Source: CAD feature listing. Evaluate the final solid. Frame: model axes, mm. A direction names the side the tool comes from. Give positions to 0.01 mm unless a question says otherwise; leave off trailing zeros. Order: outer loops, then holes, each group sorted by start corner. A loop starts at its lowest first (then second) coordinate and runs counter-clockwise, first axis right, second up.
Autodesk Inventor part; units mm, degrees
ref_plane "YZ Plane" through (0, 0, 0) normal (1, 0, 0) x (0, 1, 0)
ref_plane "XZ Plane" through (0, 0, 0) normal (0, 1, 0) x (-1, 0, 0)
ref_plane "XY Plane" through (0, 0, 0) normal (0, 0, 1) x (1, 0, 0)
sketch "Sketch1" plane through (0, 0, 0) normal (0, 1, 0) x (-1, 0, 0)
  line L0 (0, 0) -> (-85, 0)
  line L1 (-85, 0) -> (-85, -51)
  line L2 (-85, -51) -> (0, -51)
  line L3 (0, -51) -> (0, 0)
  line L4 (10, -71) -> (-95, -71)
  line L5 (-95, -71) -> (-95, 10)
  line L6 (10, 10) -> (10, -71)
  line L7 (10, 10) -> (-95, 10)
  circle A0 centre (-88, -53.5) radius 1.5
  line L8 (-42.5, -71) -> (-42.5, 10) construction
  circle A1 centre (3, -53.5) radius 1.5
  line L9 (0, -25.5) -> (-85, -25.5) construction
  circle A2 centre (-88, 2.5) radius 1.5
  circle A3 centre (3, 2.5) radius 1.5
  dimension "d0" = 85
  dimension "d1" = 51
  dimension "d2" = 20
  dimension "d3" = 10
  dimension "d4" = 10
  dimension "d13" = 2.5
  dimension "d14" = 3
  dimension "d15" = 3
  dimension "d34" = 10
extrude "Extrusion1" add sketch "Sketch1" along normal blind 5
sketch "Sketch2" plane through (95, 0, 10) normal (1, 0, 0) x (0, 0, -1)
  line L0 (68, -22.5167) -> (68, 0) construction
  line L1 (82.1908, -7.9375) -> (94.6908, 13.7132)
  line L2 (0, 0) -> (81, 0) construction
  line L3 (81, 5) -> (81, 0)
  line L4 (94.6908, 13.7132) -> (90.3607, 16.2132)
  line L5 (90.3607, 16.2132) -> (81, 0)
  line L6 (68.4427, 0) -> (82.1908, -7.9375)
  line L7 (81, 0) -> (68.4427, 0)
  point P0 (10, 0)
  dimension "d16" = 30
  dimension "d18" = 13
  dimension "d26" = 5
  dimension "d33" = 45
  dimension "d37" = 25
extrude "Extrusion2" add sketch "Sketch2" against normal blind 105
sketch "Sketch3" plane through (95, -32.5167, -58) normal (0, -0.5, -0.866) x (-1, 0, 0)
  line L0 (7.5, 46.3816) -> (97.5, 46.3816) construction
  line L1 (7.5, 43.1316) -> (97.5, 43.1316)
  line L2 (97.5, 49.6316) -> (7.5, 49.6316)
  arc A0 (7.5, 49.6316) -> (7.5, 43.1316) centre (7.5, 46.3816) ccw
  arc A1 (97.5, 43.1316) -> (97.5, 49.6316) centre (97.5, 46.3816) ccw
  line L3 (0, 53.3816) -> (105, 53.3816) construction
  point P0 (95, -0.8397)
  point P1 (52.5, 46.3816)
  point P2 (52.5, 53.3816)
  point P3 (52.5, 53.3816)
  dimension "d21" = 6.5
  dimension "d22" = 90
  dimension "d23" = 7
extrude "Extrusion3" cut sketch "Sketch3" against normal through all
sketch "Sketch4" plane through (95, 0, 10) normal (1, 0, 0) x (0, 0, -1)
  line L0 (81, 0) -> (81, 5)
  line L1 (81, 0) -> (72, 5)
  line L2 (72, 5) -> (81, 5)
  line L3 (81, 5) -> (81, 0)
  point P0 (10, 0)
  dimension "d28" = 9
extrude "Extrusion4" cut sketch "Sketch4" against normal through all
fillet "Fillet3" radius 2 3 edges at (-10, 14.9632, -82.5257) (95, 14.9632, -82.5257) (42.5, 0, -71)
fillet "Fillet4" radius 2 1 edges at (42.5, -7.9375, -72.1908)
fillet "Fillet5" radius 2 2 edges at (42.5, 5, -62) (42.5, 0, -58.4427)
fillet "Fillet6" radius 2 2 edges at (-10, 2.5, 10) (95, 2.5, 10)
equation "\"d34\" = d4"
properties part number "screen mount"
1) Section query B-B on x = 53. Output: boundary loops of the cut face in (y, z).
Checks:
outline: (-6.94, -70.46) arc R2 ccw to (-6.21, -73.19) - (4.84, -79.57) - (7.34, -75.24) - (1.7, -71.98) arc R2 cw to (0.96, -69.28) - (4.75, -62.45) arc R2 ccw to (5, -61.48) - (5, -51) - (0, -51) - (0, -57.91) arc R2 cw to (-0.27, -58.91) - close; (0, 0) - (5, 0) - (5, 10) - (0, 10) - close; (10.47, -82.82) - (13.71, -84.69) - (16.21, -80.36) - (12.97, -78.49) - close
2) Reachability of faces 1 (the face through (0, 2, -26)), 2 (the face through (42, 2, 10)), 3 (the face through (-5.75, 8.82, -79.02)), 4 (the face through (43.24, 5.84, -74.37)) from +Z, -Z, +X, -X, +Y, -Y: full face, straight path, thin tool, end or side. Return the list, or none.
Checks:
face 1: +Y, -Y
face 2: +Z, +X, -X, +Y, -Y
face 3: none
face 4: +X, -X, +Y
3) Ray query, L1, parallel to X at y = 2.25, z = -10.5; L2, parallel to Z at x = 88, y = 3.25; L3, parallel to Z at x = 88, y = 2.2. Return the intervals inside material, ascending.
Checks:
L1: x = -10 to 0, 85 to 95
L2: z = -78.65 to -72.88, -65.15 to -55, -52 to 1, 4 to 10
L3: z = -78.04 to -72.27, -67.04 to -55, -52 to 1, 4 to 10
4) First-contact query: pin 1 Ø2 at (x, y) = (17, -3.5) entering from +Z; pin 2 Ø10 at (x, y) = (13, 7) entering from -Z; pin 3 Ø1.8 at (x, z) = (88, 2.5) entering from +Y; pin 4 Ø1.5 at (x, y) = (43, 1.5) entering from -Z. Flat tips, straight axial feed; report the tip coordinate or a pass-through.
Checks:
pin 1: stops at z = -62.77
pin 2: stops at z = -83.7
pin 3: passes through
pin 4: stops at z = -78.07
5) Section query C-C on y = 3.5. Output: boundary loops of the cut face in (x, z), and give its area (3 significant figures).
Checks:
outline: (-10, -78.79) - (95, -78.79) - (95, -73.02) - (-10, -73.02) - close; (-10, -64.7) - (95, -64.7) - (95, 8) arc R2 ccw to (93, 10) - (-8, 10) arc R2 ccw to (-10, 8) - close; hole circle Ø3 at (-3, -53.5); hole circle Ø3 at (-3, 2.5); hole (0, -51) - (85, -51) - (85, 0) - (0, 0) - close; hole circle Ø3 at (88, -53.5); hole circle Ø3 at (88, 2.5)
area: 4,080 mm2
6) Section query A-A on z = -53.5. Output: boundary loops of the cut face in (x, y), and give its area (3 significant figures).
Checks:
outline: (-10, 0) - (-4.5, 0) - (-4.5, 5) - (-10, 5) - close; (-1.5, 0) - (86.5, 0) - (86.5, 5) - (-1.5, 5) - close; (89.5, 0) - (95, 0) - (95, 5) - (89.5, 5) - close
area: 495 mm2
7) Pull-direction query (X, two-part tool) for faces 5 (the face through (43.13, 6.07, -77.43)), 6 (the face through (-9.399, 14.487, -82.21)), 7 (the face through (43.24, 1.4, -77.58)); classes: +X half, -X half, draft (parallel to the pull), parting line (faces both ways), or undercut.
Checks:
face 5: undercut
face 6: -X half
face 7: draft
8) Section query D-D on z = -36.5. Output: boundary loops of the cut face in (x, y), and give its area (3 significant figures).
Checks:
outline: (-10, 0) - (0, 0) - (0, 5) - (-10, 5) - close; (85, 0) - (95, 0) - (95, 5) - (85, 5) - close
area: 100 mm2
